```python
from build123d import *

# Parameters (mm, degrees)
SKETCH1_R           = 3
BOSS_EXTRUDE1_DEPTH = 1.5875


with BuildPart() as part:
    # Sketch1 → Boss-Extrude1 (new body)
    with BuildSketch(Plane.XY):
        with BuildLine():
            Line((12.5, 0), (12.5, 210.889668604))
            ThreePointArc((12.5, 210.889668604), (7.111624908, 221.169493076), (-4.407966588, 222.586669526))
            Line((-4.407966588, 222.586669526), (-104.407966588, 184.902081679))
            ThreePointArc((-104.407966588, 184.902081679), (-111.577605538, 168.492432881), (-94.985900649, 161.754805315))
            Line((-94.985900649, 161.754805315), (-78.497504012, 168.975108381))
            Line((-78.497504012, 168.975108381), (-57.638850711, 121.341962542))
            Line((-57.638850711, 121.341962542), (-11.740989728, -4.289424229))
            ThreePointArc((-11.740989728, -4.289424229), (2.17802989, -12.308784903), (12.5, 0))
        make_face()
        with Locations((-100, 173.205080757)):
            Circle(SKETCH1_R, mode=Mode.SUBTRACT)
        with Locations((0, 210.889668604)):
            Circle(SKETCH1_R, mode=Mode.SUBTRACT)
        Circle(SKETCH1_R, mode=Mode.SUBTRACT)
        Polygon((-39.067722995, 128.792048743), (-7.5, 42.385041268), (-7.5, 200.048449538), (-61.37972985, 179.744095411), align=None, mode=Mode.SUBTRACT)
    extrude(amount=BOSS_EXTRUDE1_DEPTH)


solid = part.part
```
Geometry check sheet. Reference: the model listing, model coordinates, mm. A direction names the side the tool comes from. Coordinates: 2 decimals unless noted, no trailing zeros. Order: outer loops, then holes, each group sorted by start corner. A loop starts at its lowest first (then second) coordinate and runs counter-clockwise, first axis right, second up. Notation, with made-up numbers: (-35.75, 81.5) - (-28.75, 81.5) arc R21 ccw to (-28.75, 111.5) - close; hole circle Ø4 at (-0.5, 63). An arc over 180 degrees is marked (long way). Answer as a JSON object with one key per item and string values. Group by question number.
Item 1: Sectioned sample at A-A, the plane x = 0. Record the cut outline in (y, z).
Item 2: Scan lines: probe 1 along Y at (x, z) = (-100, 1.15); probe 2 along X at (y, z) = (79, 1.45); probe 3 along X at (y, z) = (74.5, 0.8). Record each from-to range of solid material in increasing order.
Item 3: Sectioned sample at D-D, the plane x = -25. Record the cut outline in (y, z), and give its area (3 significant figures).
Item 4: Tool access check on faces 4 (the face through (-86.857, 165.314, 0.783)), 5 (the face through (-53.708, 204.008, 0.783)), 6 (the face through (-23.505, 86.193, 0.783)). Record the directions out of +Z, -Z, +X, -X, +Y, -Y that give a thin tool (end or side, any length) a straight path to the whole face; none if there is none.
Item 5: Draft check along Y on faces 1 (the face through (-68, 145, 1)), 2 (the face through (-111.7, 168.8, 0.8)), 3 (the face through (-50.38, 154.62, 0.78)). Enter one of: +Y half, -Y half, draft (parallel to the pull), parting line (faces both ways), or undercut.
Item 6: Depth check by flat-ended pin: pin 1 Ø5 at (x, y) = (0, 210.89) entering from -Z. Enter the tip coordinate at first touch or a pass-through.
Item 7: Sectioned sample at C-C, the plane z = 0.85. Record the cut outline in (x, y), and give its area (3 significant figures).
Item 8: Sectioned sample at B-B, the plane y = 84.5. Record the cut outline in (x, z), and give its area (3 significant figures).
Resolved:
{
 "1": {"outline": "(-12.5, 0) - (-3, 0) - (-3, 1.59) - (-12.5, 1.59) - close; (3, 0) - (207.89, 0) - (207.89, 1.59) - (3, 1.59) - close; (213.89, 0) - (223.39, 0) - (223.39, 1.59) - (213.89, 1.59) - close"},
 "2": {"probe 1": "160.71 to 170.21, 176.21 to 186.56", "probe 2": "-42.17 to -20.88, -7.5 to 12.5", "probe 3": "-40.53 to -19.23, -7.5 to 12.5"},
 "3": {"outline": "(32, 0) - (90.29, 0) - (90.29, 1.59) - (32, 1.59) - close; (193.45, 0) - (214.83, 0) - (214.83, 1.59) - (193.45, 1.59) - close", "area": "126 mm^2"},
 "4": {"face 4": "+Z, -Z, -Y", "face 5": "+Z, -Z, -X, +Y", "face 6": "+Z, -Z"},
 "5": {"face 1": "-Y half", "face 2": "parting line", "face 3": "undercut"},
 "6": {"pin 1": "through"},
 "7": {"outline": "(-104.41, 184.9) arc R12.5 ccw (long way) to (-94.99, 161.75) - (-78.5, 168.98) - (-57.64, 121.34) - (-11.74, -4.29) arc R12.5 ccw to (12.5, 0) - (12.5, 210.89) arc R12.5 ccw to (-4.41, 222.59) - close; hole circle Ø6 at (-100, 173.21); hole (-61.38, 179.74) - (-39.07, 128.79) - (-7.5, 42.39) - (-7.5, 200.05) - close; hole circle Ø6 at (0, 0); hole circle Ø6 at (0, 210.89)", "area": "10,400 mm^2"},
 "8": {"outline": "(-44.18, 0) - (-22.89, 0) - (-22.89, 1.59) - (-44.18, 1.59) - close; (-7.5, 0) - (12.5, 0) - (12.5, 1.59) - (-7.5, 1.59) - close", "area": "65.6 mm^2"}
}
